Could you check a few things on this drawing? It's one solid part, dimensions in mm from its lowest x, y, z. A direction names the side the tool comes from. Round coordinates to 2 decimals unless told otherwise and drop trailing zeros. Write each loop counter-clockwise with the first axis right and the second up, starting at its lowest first coordinate (ties: lowest second). Pieces come first, ordered by that corner, then holes. Notation, with made-up numbers: (35, -5.5) -> (74, -5.5) arc R25 cw to (74, 33.5) -> close; hole circle Ø7 at (-15.75, -34). An arc over 180 degrees is marked (long way). Answer as CSV lines item,"result".
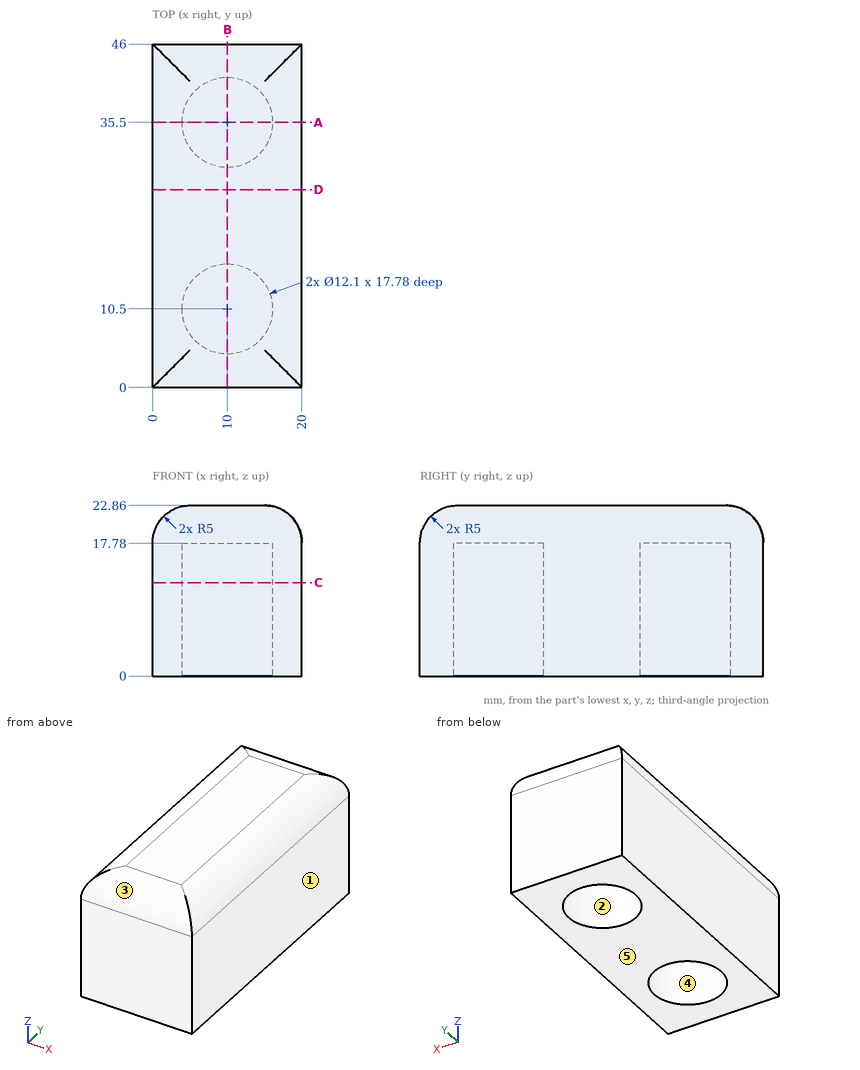
1. For pin 1 Ø3.5 at (x, y) = (10, 11) entering from -Z; pin 2 Ø2 at (x, z) = (12.5, 19.5) entering from +Y, each with a flat end and sliding along its axis, tell me the tip position at first contact or that it passes through.
Numbers:
pin 1,"stops at z = 17.78"
pin 2,"stops at y = 45.96"
2. Suppose I cut it at A-A on y = 35.5. Please give me the cut outline in (x, z).
Numbers:
outline,"(0, 0) -> (3.95, 0) -> (3.95, 17.78) -> (16.05, 17.78) -> (16.05, 0) -> (20, 0) -> (20, 17.86) arc R5 ccw to (15, 22.86) -> (5, 22.86) arc R5 ccw to (0, 17.86) -> close"
3. Suppose I cut it at D-D on y = 26.5. Please give me the cut outline in (x, z), and give its area (3 significant figures).
Numbers:
outline,"(0, 0) -> (20, 0) -> (20, 17.86) arc R5 ccw to (15, 22.86) -> (5, 22.86) arc R5 ccw to (0, 17.86) -> close"
area,"446 mm^2"
4. If I drill on line 1 (Y direction, x = 10, z = 8.25); line 2 (Y direction, x = 12.5, z = 14.5); line 3 (Z direction, x = 10.25, y = 34), over which ranges is the centre line in solid material (lowest first)?
Numbers:
line 1,"y = 0 to 4.45, 16.55 to 29.45, 41.55 to 46"
line 2,"y = 0 to 4.99, 16.01 to 29.99, 41.01 to 46"
line 3,"z = 17.78 to 22.86"
5. Suppose I cut it at C-C on z = 12.5. Please give me the cut outline in (x, y).
Numbers:
outline,"(0, 0) -> (20, 0) -> (20, 46) -> (0, 46) -> close; hole circle Ø12.1 at (10, 10.5); hole circle Ø12.1 at (10, 35.5)"
6. Suppose I cut it at B-B on x = 10. Please give me the cut outline in (y, z).
Numbers:
outline,"(0, 0) -> (4.45, 0) -> (4.45, 17.78) -> (16.55, 17.78) -> (16.55, 0) -> (29.45, 0) -> (29.45, 17.78) -> (41.55, 17.78) -> (41.55, 0) -> (46, 0) -> (46, 17.86) arc R5 ccw to (41, 22.86) -> (5, 22.86) arc R5 ccw to (0, 17.86) -> close"
7. If we mould it in two halves opening along X, with no side actions, what happens to the marked faces 1, 2 and 3? For each: released by +X, released by -X, zero draft, split by the parting line, or undercut.
Numbers:
face 1,"released by +X"
face 2,"undercut"
face 3,"zero draft"
8. On a 3-axis mill with a long thin cutter (end or side, diameter ignored), from which of +Z, -Z, +X, -X, +Y, -Y can I reach the whole of each face in a straight line? I mean the marked faces 4 and 5. Say none if no direction works.
Numbers:
face 4,"-Z"
face 5,"-Z, +X, -X, +Y, -Y"
